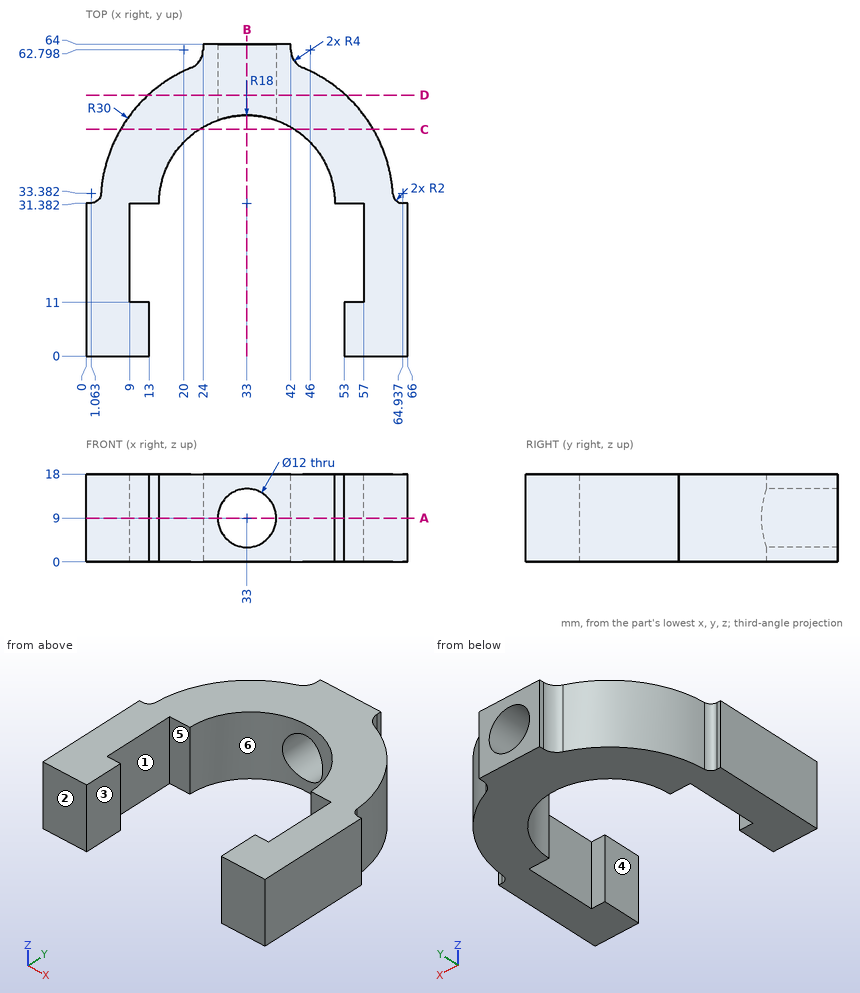
Could you check a few things on this drawing? It's one solid part, dimensions in mm from its lowest x, y, z. A direction names the side the tool comes from. Coordinates: 2 decimals unless noted, no trailing zeros. Order: outer loops, then holes, each group sorted by start corner. A loop starts at its lowest first (then second) coordinate and runs counter-clockwise, first axis right, second up.
1. If we section it at C-C (y = 46.5): Please give me the cut outline in (x, z).
2. I need wall thicknesses on line 1 (X direction, y = 22.5, z = 16); line 2 (Z direction, x = 33, y = 54.5); line 3 (X direction, y = 7, z = 15). Which ranges of each line are inside material? Lowest first, please.
3. For the marked faces 1, 2 and 3, which set-ups out of +Z, -Z, +X, -X, +Y, -Y let a thin tool reach every point of the face, with its end or its side?
4. I'm going to push flat-ended pins straight in: pin 1 (9 mm diameter, centred on y = 19, z = 6, fed in from -X); pin 2 (1 mm diameter, centred on y = 63.5, z = 8, fed in from -X); pin 3 (10 mm diameter, centred on x = 49.5, z = 13, fed in from +Y); pin 4 (8 mm diameter, centred on x = 54, z = 15, fed in from +Y). Where does each tip first touch, or does it pass through?
5. If we section it at A-A (z = 9): Please give me the cut outline in (x, y).
6. Thinking about a two-plate mould opening in Y: for the marked faces 4, 5 and 6, which applies, +Y half, -Y half, draft (parallel to the pull), parting line (faces both ways), or undercut?
7. If we section it at B-B (x = 33): Please give me the cut outline in (y, z).
8. If we section it at D-D (y = 53.5): Please give me the cut outline in (x, z).
Entries:
1. outline: (7.09, 0) - (23.23, 0) - (23.23, 18) - (7.09, 18) - close; (42.77, 0) - (58.91, 0) - (58.91, 18) - (42.77, 18) - close
2. line 1: x = 0 to 9, 57 to 66
2. line 2: z = 0 to 3, 15 to 18
2. line 3: x = 0 to 13, 53 to 66
3. face 1: +Z, -Z
3. face 2: +Z, -Z, +X, -X, -Y
3. face 3: +Z, -Z, -Y
4. pin 1: stops at x = 0
4. pin 2: stops at x = 24
4. pin 3: stops at y = 59.09
4. pin 4: stops at y = 56.1
5. outline: (0, 0) - (13, 0) - (13, 11) - (9, 11) - (9, 31.38) - (15, 31.38) arc R18 cw to (27, 48.35) - (27, 64) - (24, 64) - (24, 62.8) arc R4 cw to (21.53, 59.1) arc R30 ccw to (3.06, 33.26) arc R2 cw to (1.06, 31.38) - (0, 31.38) - close; (39, 48.35) arc R18 cw to (51, 31.38) - (57, 31.38) - (57, 11) - (53, 11) - (53, 0) - (66, 0) - (66, 31.38) - (64.94, 31.38) arc R2 cw to (62.94, 33.26) arc R30 ccw to (44.47, 59.1) arc R4 cw to (42, 62.8) - (42, 64) - (39, 64) - close
6. face 4: draft
6. face 5: undercut
6. face 6: -Y half
7. outline: (49.38, 0) - (64, 0) - (64, 3) - (49.38, 3) - close; (49.38, 15) - (64, 15) - (64, 18) - (49.38, 18) - close
8. outline: (12.73, 0) - (53.27, 0) - (53.27, 18) - (12.73, 18) - close; hole circle Ø12 at (33, 9)
